```python
from build123d import *

# Parameters (mm, degrees)
BOSS_EXTRUDE1_DEPTH = 2
SKETCH2_R           = 3.05
SKETCH2_R_2         = 4.740417633
CUT_EXTRUDE1_DEPTH  = 10


with BuildPart() as part:
    # Sketch1 → Boss-Extrude1 (new body)
    with BuildSketch(Plane.XY):
        Polygon((192.039285274, 88.983833718), (201.963048499, 79.060070494), (192.039285274, -11.016166282), (-18.008037477, -11.016166282), (-63.036951501, 54.472600305), (-18.008037477, 79.060070494), (131.67120814, 79.060070494), (131.67120814, 88.983833718), align=None)
    extrude(amount=BOSS_EXTRUDE1_DEPTH)

    # Sketch2 → Cut-Extrude1 (cut)
    with BuildSketch(Plane.XY.offset(2)):
        with Locations((49.886677935, 34.46755227)):
            Circle(SKETCH2_R)
        with Locations((47.903695827, 8.119584274)):
            Circle(SKETCH2_R_2)
    extrude(amount=-CUT_EXTRUDE1_DEPTH, mode=Mode.SUBTRACT)


solid = part.part
```
Could you check a few things on this model? Use its own coordinates, in mm. Give positions to 0.01 mm unless a question says otherwise; leave off trailing zeros. Write each loop counter-clockwise with the first axis right and the second up, starting at its lowest first coordinate (ties: lowest second). Pieces come first, ordered by that corner, then holes. Notation, with made-up numbers: (-29, -21) - (25, -21) arc R16 ccw to (25, -4) - close; hole circle Ø6 at (9, -16.75). An arc over 180 degrees is marked (long way). One line per item, written item: value. Start each with the question number.
Item 1: I'm going to push flat-ended pins straight in: pin 1 (3.5 mm diameter, centred on x = 49.89, y = 34.47, fed in from -Z); pin 2 (1 mm diameter, centred on y = 85, z = 1, fed in from -X). Where does each tip first touch, or does it pass through?
Item 2: Imagine slicing it at C-C, the plane y = 67. List the corners of the cut face in (x, z) for me, and give its area (3 significant figures).
Item 3: Please list where these lines run through material, in increasing order: line 1 (Y direction, x = 115, z = 0.65); line 2 (X direction, y = 12, z = 1.4) (3 decimals); line 3 (X direction, y = 7, z = 1.15). Write a range as from..to.
Item 4: Imagine slicing it at A-A, the plane x = 6.5. List the corners of the cut face in (y, z) for me.
Item 5: If we mould it in two halves opening along Y, with no side actions, what happens to faces 1 (the face through (51.526, 37.039, 1.014)), 2 (the face through (197.07, 34.65, 0.99)), 3 (the face through (71, 40, 2))? For each: +Y half, -Y half, draft (parallel to the pull), parting line (faces both ways), or undercut.
Item 6: Imagine slicing it at B-B, the plane z = 1.7. List the corners of the cut face in (x, y) for me.
Geometry says:
1. pin 1: through
1. pin 2: x = 131.67
2. outline: (-40.09, 0) - (200.63, 0) - (200.63, 2) - (-40.09, 2) - close
2. area: 481 mm^2
3. line 1: -11.02..79.06
3. line 2: -33.834..45.181, 50.627..194.575
3. line 3: -30.4..43.3, 52.51..194.02
4. outline: (-11.02, 0) - (79.06, 0) - (79.06, 2) - (-11.02, 2) - close
5. face 1: undercut
5. face 2: -Y half
5. face 3: draft
6. outline: (-63.04, 54.47) - (-18.01, -11.02) - (192.04, -11.02) - (201.96, 79.06) - (192.04, 88.98) - (131.67, 88.98) - (131.67, 79.06) - (-18.01, 79.06) - close; hole circle Ø9.48 at (47.9, 8.12); hole circle Ø6.1 at (49.89, 34.47)
